CAD build for the part. Positions are in the model's coordinates, mm. A direction names the side the tool comes from. Round coordinates to 2 decimals unless told otherwise and drop trailing zeros. Order: outer loops, then holes, each group sorted by start corner. A loop starts at its lowest first (then second) coordinate and runs counter-clockwise, first axis right, second up. Notation, with made-up numbers: M 88,51 L 97,51 A20 cw 97,70 Z; hole C -26,75.5 d9. An arc over 180 degrees is marked long. Put each result on its own line as item: value.
```python
from build123d import *

# Parameters (mm, degrees)
SKETCH2_W               = 25.203593645
SKETCH2_H               = 76.2
SKETCH2_W_2             = 66.311902543
SKETCH2_H_2             = 95.27897735
SKETCH3_W               = 25.4
SKETCH3_H               = 12.7
CUT_EXTRUDE1_DEPTH      = 373.934318072
CUT_EXTRUDE2_DEPTH      = 328.295564346
CUT_EXTRUDE2_DEPTH_BACK = 328.295564346
SKETCH4_W               = 25.196915696
SKETCH4_H               = 12.7
SKETCH5_R               = 50.8
CUT_EXTRUDE3_DEPTH      = 557.821446487
SKETCH6_R               = 6.35
CUT_EXTRUDE4_DEPTH      = 25.4
CUT_EXTRUDE5_START      = -25.4
SKETCH7_R               = 6.35
CUT_EXTRUDE5_DEPTH      = 25.4
SKETCH8_R               = 76.2
CUT_EXTRUDE8_DEPTH      = 38.1


with BuildPart() as part:
    # Sketch2 → Revolve1 (revolve)
    with BuildSketch(Plane(origin=(0, 0, 0), x_dir=(1, 0, 0), z_dir=(0, 1, 0)), mode=Mode.PRIVATE) as revolve1_sk:
        Polygon((-266.7, 82.55), (-266.7, 0), (-215.9, 0), (-215.9, 76.2), (-215.9, 82.55), align=None)
        with Locations((-203.298203177, 38.1)):
            Rectangle(SKETCH2_W, SKETCH2_H)
        Polygon((-190.696406355, 76.2), (-190.696406355, 0), (88.703593645, 0), (88.703593645, 95.27897735), (88.703593645, 101.6), (-190.696406355, 101.6), align=None)
        with Locations((121.859544917, 47.639488675)):
            Rectangle(SKETCH2_W_2, SKETCH2_H_2)
        Polygon((155.015496188, 95.27897735), (155.015496188, 0), (166.010986047, 0), (166.010986047, 95.27897735), (160.513241117, 89.781232421), align=None)
        Polygon((166.010986047, 95.27897735), (166.010986047, 0), (177.006475906, 0), (177.006475906, 95.27897735), (171.508730976, 89.781232421), align=None)
        Polygon((177.006475906, 95.27897735), (177.006475906, 0), (183.724405052, 0), (183.724405052, 101.62897735), (183.724405052, 112.992396356), (177.006475906, 112.992396356), align=None)
        Polygon((183.724405052, 101.62897735), (183.724405052, 0), (266.7, 0), (266.7, 82.55), (242.364065099, 82.55), align=None)
    revolve(revolve1_sk.sketch.rotate(Axis((-266.7, 0, 0), (1, 0, 0)), 180), axis=Axis((-266.7, 0, 0), (1, 0, 0)))

    # Sketch3 → Cut-Extrude1 (cut, through all)
    with BuildSketch(Plane(origin=(0, 121.92, 0), x_dir=(1, 0, 0), z_dir=(0, 1, 0))):
        with Locations((212.824212149, 43.140904216)):
            Rectangle(SKETCH3_W, SKETCH3_H)
        with Locations((212.824212149, -33.059095784)):
            Rectangle(SKETCH3_W, SKETCH3_H)
    extrude(amount=-CUT_EXTRUDE1_DEPTH, mode=Mode.SUBTRACT)

    # Sketch4 → Cut-Extrude2 (cut, two sides: drawn at the far end of the back side and taken through both)
    with BuildSketch(Plane(origin=(0, 0, 39.409095784), x_dir=(-1, 0, 0), z_dir=(0, 0, -1)).offset(-CUT_EXTRUDE2_DEPTH_BACK)):
        with Locations((-212.925754301, 38.015203285)):
            Rectangle(SKETCH4_W, SKETCH4_H)
        with Locations((-212.925754301, -38.184796715)):
            Rectangle(SKETCH4_W, SKETCH4_H)
    extrude(amount=CUT_EXTRUDE2_DEPTH + CUT_EXTRUDE2_DEPTH_BACK, mode=Mode.SUBTRACT)

    # Sketch5 → Cut-Extrude3 (cut, through all)
    with BuildSketch(Plane.ZY.offset(266.7)):
        Circle(SKETCH5_R)
    extrude(amount=-CUT_EXTRUDE3_DEPTH, mode=Mode.SUBTRACT)

    # Sketch6 → Cut-Extrude4 (cut)
    with BuildSketch(Plane.ZY.offset(266.7)):
        with Locations((0, 66.675)):
            Circle(SKETCH6_R)
        with Locations((47.146344636, 47.146344636)):
            Circle(SKETCH6_R)
        with Locations((66.675, 0)):
            Circle(SKETCH6_R)
        with Locations((47.146344636, -47.146344636)):
            Circle(SKETCH6_R)
        with Locations((0, -66.675)):
            Circle(SKETCH6_R)
        with Locations((-47.146344636, -47.146344636)):
            Circle(SKETCH6_R)
        with Locations((-66.675, 0)):
            Circle(SKETCH6_R)
        with Locations((-47.146344636, 47.146344636)):
            Circle(SKETCH6_R)
    extrude(amount=-CUT_EXTRUDE4_DEPTH, mode=Mode.SUBTRACT)

    # Sketch7 → Cut-Extrude5 (cut)
    with BuildSketch(Plane(origin=(266.7, 0, 0), x_dir=(0, 0, -1), z_dir=(1, 0, 0)).offset(CUT_EXTRUDE5_START)):
        with Locations(Location((0, 66.675, 0), (0, 0, 180))):
            Circle(SKETCH7_R)
        with Locations(Location((47.146344636, 47.146344636, 0), (0, 0, 180))):
            Circle(SKETCH7_R)
        with Locations(Location((66.675, 0, 0), (0, 0, 180))):
            Circle(SKETCH7_R)
        with Locations(Location((47.146344636, -47.146344636, 0), (0, 0, 180))):
            Circle(SKETCH7_R)
        with Locations(Location((0, -66.675, 0), (0, 0, 180))):
            Circle(SKETCH7_R)
        with Locations(Location((-47.146344636, -47.146344636, 0), (0, 0, 180))):
            Circle(SKETCH7_R)
        with Locations(Location((-66.675, 0, 0), (0, 0, 180))):
            Circle(SKETCH7_R)
        with Locations(Location((-47.146344636, 47.146344636, 0), (0, 0, 180))):
            Circle(SKETCH7_R)
    extrude(amount=CUT_EXTRUDE5_DEPTH, mode=Mode.SUBTRACT)

    # Sketch8 → Cut-Extrude8 (cut)
    with BuildSketch(Plane(origin=(0, 101.6, 0), x_dir=(1, 0, 0), z_dir=(0, 1, 0))):
        with Locations(Location((0, 0, 0), (0, 0, 270))):
            Circle(SKETCH8_R)
    extrude(amount=-CUT_EXTRUDE8_DEPTH, mode=Mode.SUBTRACT)


solid = part.part
```
Item 1: Band-saw the part on C-C on z = 67.5. State how many separate pieces and enclosed holes the cut face has, and give its area (3 significant figures).
Answers below:
separate pieces: 1
enclosed holes: 2
area: 69,400 mm²
Item 2: Band-saw the part on B-B on x = 18. Give the cut face in (y, z).
Answers below:
outline: M 63.5,-74.04 L 63.5,74.04 L 69.57,74.04 A101.6 ccw long 69.57,-74.04 Z; hole C 0,0 d101.6
Item 3: Tool access for faces 1 (the cylindrical face through (-254.18, 0.28, -73.02)), 2 (the cylindrical face through (253.82, -1.91, 72.73)), 3 (the flat face through (225.524, -44, 45)), 4 (the flat face through (213, -44.535, -31)), 5 (the flat face through (213, -68, -36.791)): list every direction of +Z, -Z, +X, -X, +Y, -Y with a clear straight run to the whole face (end or side of a thin tool).
Answers below:
face 1: -X
face 2: +X
face 3: none
face 4: +Z, -Z
face 5: +Y, -Y
Item 4: Probe line 1 along Z through (x, y) = (204, -74); line 2 along X through (y, z) = (60.5, 36); line 3 along Y through (x, z) = (87, -0.5). List the from-to ranges inside material, lowest first. Write a range as [from, to].
Answers below:
line 1: [-59.62, -49.49], [-36.79, 26.71], [39.41, 59.62]
line 2: [-266.7, 200.12], [225.52, 266.7]
line 3: [-101.6, -50.8], [50.8, 101.6]
Item 5: Pin check, flat tips, straight feed: P1, Ø12.5, axis at x = 213, z = -64, coming from the -Y side; P2, Ø20.5, axis at y = -47.15, z = -47.15, coming from the +X side; P3, Ø5, axis at x = 134, z = -77.5, coming from the +Y side; P4, Ø10, axis at y = 0, z = -66.675, coming from the +X side. Stop position of each tip, or through.
Answers below:
P1: y = -72.39
P2: x = 266.7
P3: y = 58.76
P4: x = 241.3
Item 6: Band-saw the part on A-A on x = -167. Give the cut face in (y, z).
Answers below:
outline: C 0,0 d203.2; hole C 0,0 d101.6
Item 7: Mould opens along X. For faces 6 (the flat face through (-241.3, 47, -47)), 7 (the conical face through (238.7, -3.68, -83.66)), 8 (the cylindrical face through (75.55, 78.59, -9.92)), 9 (the flat face through (213, 44.365, -31)) say: pulls with the +X half, pulls with the -X half, needs draft (parallel to the pull), parting line crosses it, or undercut.
Answers below:
face 6: pulls with the -X half
face 7: pulls with the +X half
face 8: undercut
face 9: undercut
